For this review, take the finished solid that the model builds, in its own axes (mm). A direction names the side the tool comes from. Give positions to 0.01 mm unless a question says otherwise; leave off trailing zeros. Loops run counter-clockwise (first coordinate to the right, second up) from the corner with the lowest first, then second, coordinate; pieces in that order, holes last. Notation, with made-up numbers: (67.25, 77) -> (114.25, 77) arc R16 cw to (114.25, 102) -> close; hole circle Ø8 at (26.5, 46.25). An arc over 180 degrees is marked (long way). Answer as CSV lines item,"result". Start each with the question number.
Item 1: Clearance check with flat-ended pins moving along their axes: P1, Ø22.5, axis at y = 138, z = -14, coming from the -X side; P2, Ø1.5, axis at x = -89.5, y = 137, coming from the +Z side; P3, Ø4, axis at x = -50, z = 23, coming from the +Y side. State where each tip first meets the part, or that it passes through.
Item 2: For L1, parallel to X at y = 134, z = -32; L2, parallel to X at y = 84, z = 2; L3, parallel to Z at x = -129, y = 153, list the stretches that pass through material, from the lowest coordinate up. Write a range as from..to.
Item 3: Add section C-C on x = -72.5. State the section outline as (y, z) points.
Item 4: Machinability: for faces 1 (the face through (25.77, 129.957, -0.651)), 2 (the face through (52.271, 125, 0)), 3 (the face through (-157.379, 129.957, -0.651)), which of the approach directions +Z, -Z, +X, -X, +Y, -Y give a long, thin tool a straight path to every point of the face, cutting with its end or side? Answer none if there is none.
Item 5: Add section D-D on x = -145. State the section outline as (y, z) points, plus the area to 3 significant figures.
```python
from build123d import *

# Parameters (mm, degrees)
SKETCH3_R                = 5
BOSS_EXTRUDE1_DEPTH      = 50
BOSS_EXTRUDE1_DEPTH_BACK = 185


with BuildPart() as part:
    # Sketch2 → Revolve1 (revolve)
    with BuildSketch(Plane.XY):
        with BuildLine():
            Line((-126.767029403, 81.676904789), (-78.228933631, 79.25))
            ThreePointArc((-78.228933631, 79.25), (-60.619483805, 77.84878425), (-43.123035518, 75.413537626))
            ThreePointArc((-43.123035518, 75.413537626), (-41.060447751, 74.831340884), (-39.169286378, 73.823010577))
            ThreePointArc((-39.169286378, 73.823010577), (-35.312933401, 70.206346657), (-32.754159078, 65.579858771))
            Line((-32.754159078, 65.579858771), (-32.056761325, 63.663774193))
            ThreePointArc((-32.056761325, 63.663774193), (-31.860334358, 63.066262055), (-31.701859109, 62.457583237))
            ThreePointArc((-31.701859109, 62.457583237), (-26.081952508, 53.496427146), (-16.098933631, 50))
            Line((-16.098933631, 50), (-16, 50))
            ThreePointArc((-16, 50), (-4.686291501, 54.686291501), (0, 66))
            Line((0, 66), (0, 78.5))
            Line((0, 78.5), (0, 125))
            Line((0, 125), (-132.728933631, 125))
            Line((-132.728933631, 125), (-132.728933631, 97.760533906))
            Line((-132.728933631, 97.760533906), (-132.728933631, 87.760533906))
            ThreePointArc((-132.728933631, 87.760533906), (-132.538632462, 86.803825325), (-131.996700584, 85.992766953))
            Line((-131.996700584, 85.992766953), (-128.409952314, 82.406018683))
            ThreePointArc((-128.409952314, 82.406018683), (-127.656283908, 81.888702675), (-126.767029403, 81.676904789))
        make_face()
    revolve(axis=Axis((0, 125, 0), (-1, 0, 0)))

    # Sketch3 → Boss-Extrude1 (add, two sides)
    with BuildSketch(Plane.ZY.offset(132.728933631)) as boss_extrude1_sk:
        with Locations((0, 125)):
            Circle(SKETCH3_R)
    extrude(amount=BOSS_EXTRUDE1_DEPTH)
    extrude(boss_extrude1_sk.sketch, amount=-BOSS_EXTRUDE1_DEPTH_BACK)


solid = part.part
```
Computed values:
1,P1,"x = -132.73"
1,P2,"z = 43.77"
1,P3,"y = 168.78"
2,L1,"-132.73..0"
2,L2,"-129.96..0"
2,L3,"-31.31..31.31"
3,outline,"circle Ø92.18 at (125, 0)"
4,face 1,"+X"
4,face 2,"+Z, -Z, +X, +Y, -Y"
4,face 3,"-X"
5,outline,"circle Ø10 at (125, 0)"
5,area,"78.5 mm²"
